CAD build for the part. Positions are in the model's coordinates, mm. A direction names the side the tool comes from. Give positions to 0.01 mm unless a question says otherwise; leave off trailing zeros. Loops run counter-clockwise (first coordinate to the right, second up) from the corner with the lowest first, then second, coordinate; pieces in that order, holes last. Notation, with made-up numbers: (-0.75, 76) - (42.25, 76) arc R33 cw to (42.25, 109) - close; hole circle Ø7 at (74, 21). An arc over 180 degrees is marked (long way). Return JSON: item names as keys, results as strings.
from build123d import *

# Parameters (mm, degrees)
BOSS_EXTRUDE1_DEPTH       = 35
BOSS_EXTRUDE1_DEPTH_BACK  = 35
SKETCH2_W                 = 70
SKETCH2_H                 = 70
BOSS_EXTRUDE2_DEPTH       = 32.5
BOSS_EXTRUDE2_DEPTH_BACK  = 32.5
SKETCH3_W                 = 10
SKETCH3_H                 = 65
BOSS_EXTRUDE10_DEPTH      = 32.5
BOSS_EXTRUDE10_DEPTH_BACK = 32.5
SKETCH20_W                = 10
SKETCH20_H                = 65
SKETCH6_W                 = 65
SKETCH6_H                 = 65
BOSS_EXTRUDE4_DEPTH       = 10
BOSS_EXTRUDE6_DEPTH       = 32.5
BOSS_EXTRUDE6_DEPTH_BACK  = 32.5
SKETCH12_W                = 66.54355119
SKETCH12_H                = 10
SKETCH13_W                = 15
SKETCH13_H                = 15.886543597
BOSS_EXTRUDE7_DEPTH       = 19
BOSS_EXTRUDE7_DEPTH_BACK  = 19
SKETCH16_W                = 15.65
SKETCH16_H                = 15
BOSS_EXTRUDE14_DEPTH      = 65
CUT_EXTRUDE2_REACH        = 292.31
SKETCH25_R                = 3.001207037
SKETCH25_R_2              = 3
CUT_EXTRUDE3_REACH        = 292.31


with BuildPart() as part:
    # Sketch2 → Boss-Extrude1 (new, two sides: drawn at the far end of the back side and taken through both)
    with BuildSketch(Plane.XY.offset(-BOSS_EXTRUDE1_DEPTH_BACK)):
        Rectangle(SKETCH2_W, SKETCH2_H)
    extrude(amount=BOSS_EXTRUDE1_DEPTH + BOSS_EXTRUDE1_DEPTH_BACK)

    # Sketch3 → Boss-Extrude2 (add, two sides: drawn at the far end of the back side and taken through both)
    with BuildSketch(Plane.XY.offset(-BOSS_EXTRUDE2_DEPTH_BACK)):
        with Locations((40, 0)):
            Rectangle(SKETCH3_W, SKETCH3_H)
    extrude(amount=BOSS_EXTRUDE2_DEPTH + BOSS_EXTRUDE2_DEPTH_BACK)

    # Sketch20 → Boss-Extrude10 (add, two sides: drawn at the far end of the back side and taken through both)
    with BuildSketch(Plane.XY.offset(-BOSS_EXTRUDE10_DEPTH_BACK)):
        with Locations((-40, 0)):
            Rectangle(SKETCH20_W, SKETCH20_H)
    extrude(amount=BOSS_EXTRUDE10_DEPTH + BOSS_EXTRUDE10_DEPTH_BACK)

    # Sketch4 → Revolve1 (revolve)
    with BuildSketch(Plane.XY, mode=Mode.PRIVATE) as revolve1_sk:
        Polygon((45, 28), (59.607985015, 28), (59.607985015, 29.5), (67.607985015, 29.5), (74.107985015, 26.85697368), (74.107985015, 0), (45, 0), align=None)
    revolve(revolve1_sk.sketch.rotate(Axis((126.079032841, 0, 0), (-1, 0, 0)), 90), axis=Axis((126.079032841, 0, 0), (-1, 0, 0)))

    # Sketch5 → Revolve2 (revolve)
    with BuildSketch(Plane.XY, mode=Mode.PRIVATE) as revolve2_sk:
        Polygon((74.107985015, 25), (174.107985015, 0), (74.107985015, 0), align=None)
    revolve(revolve2_sk.sketch.rotate(Axis((0, 0, 0), (1, 0, 0)), 90), axis=Axis((0, 0, 0), (1, 0, 0)))

    # Sketch11 → Revolve4 (revolve)
    with BuildSketch(Plane.XY, mode=Mode.PRIVATE) as revolve4_sk:
        Polygon((-45, 28), (-57.201085702, 28), (-57.201085702, 31.288573188), (-80.147769564, 31.288573188), (-80.147769564, 30.339674147), (-106.73557157, 30.339674147), (-106.73557157, 28), (-148.804473643, 28), (-162.901896786, 23.768340348), (-162.901896786, 13.75175022), (-172.176517275, 13.75175022), (-172.176517275, 11.711333713), (-294.985996393, 11.711333713), (-294.985996393, 0), (-45, 0), align=None)
    revolve(revolve4_sk.sketch.rotate(Axis((0, 0, 0), (-1, 0, 0)), 90), axis=Axis((0, 0, 0), (-1, 0, 0)))

    # Sketch6 → Boss-Extrude4 (add)
    with BuildSketch(Plane.XZ.offset(35)):
        Rectangle(SKETCH6_W, SKETCH6_H)
    extrude(amount=BOSS_EXTRUDE4_DEPTH)

    # Sketch12 → Boss-Extrude6 (add, two sides: drawn at the far end of the back side and taken through both)
    with BuildSketch(Plane.XY.offset(-BOSS_EXTRUDE6_DEPTH_BACK)):
        with Locations((0, 40)):
            Rectangle(SKETCH12_W, SKETCH12_H)
    extrude(amount=BOSS_EXTRUDE6_DEPTH + BOSS_EXTRUDE6_DEPTH_BACK)

    # Sketch13 → Revolve5 (revolve)
    with BuildSketch(Plane.XY, mode=Mode.PRIVATE) as revolve5_sk:
        with Locations((7.5, 52.943271799)):
            Rectangle(SKETCH13_W, SKETCH13_H)
    revolve(revolve5_sk.sketch.rotate(Axis((0, 0, 0), (0, 1, 0)), 90), axis=Axis((0, 0, 0), (0, 1, 0)))

    # Sketch14 → Boss-Extrude7 (add, two sides: drawn at the far end of the back side and taken through both)
    with BuildSketch(Plane.XY.offset(-BOSS_EXTRUDE7_DEPTH_BACK)):
        Polygon((-19, 60.650657798), (19, 60.650657798), (19, 66.650657798), (-7.5, 93.150657798), (-19, 93.150657798), align=None)
    extrude(amount=BOSS_EXTRUDE7_DEPTH + BOSS_EXTRUDE7_DEPTH_BACK)

    # Sketch15 → Revolve6 (revolve)
    with BuildSketch(Plane.XY):
        Polygon((-19, 91.400657798), (-25, 91.400657798), (-25, 82.400657798), (-33.5, 82.400657798), (-33.5, 88.400657798), (-71.5, 88.400657798), (-71.5, 86.900657798), (-79.5, 86.900657798), (-79.5, 76.900657798), (-19, 76.900657798), align=None)
    revolve(axis=Axis((23.08157289, 76.900657798, 0), (-1, 0, 0)))

    # Sketch16 → Revolve7 (revolve)
    with BuildSketch(Plane.XY):
        with Locations((-52.825, 7.5)):
            Rectangle(SKETCH16_W, SKETCH16_H)
    revolve(axis=Axis((0, 0, 0), (-1, 0, 0)))

    # Sketch24 → Boss-Extrude14 (add)
    with BuildSketch(Plane.XY.offset(32.5)):
        Polygon((-32.5, -45), (24.068542495, -101.568542495), (31.139610307, -94.497474683), (-18.357864376, -45), align=None)
    extrude(amount=-BOSS_EXTRUDE14_DEPTH)

    # Sketch25 → Cut-Extrude2 (cut, up to next)
    with BuildSketch(Plane(origin=(-38.75, -38.75, 0), x_dir=(0, 0, 1), z_dir=(-0.7071067811865438, -0.7071067811865512, 0)), mode=Mode.PRIVATE) as cut_extrude2_sk1:
        with Locations(Location((0, -83.838834765, 0), (0, 0, 270))):
            Circle(SKETCH25_R)
    cut_extrude2_tool1 = extrude(cut_extrude2_sk1.sketch, amount=-CUT_EXTRUDE2_REACH, mode=Mode.PRIVATE) & part.part
    # Sketch25 → Cut-Extrude2 (cut, up to next)
    with BuildSketch(Plane(origin=(-38.75, -38.75, 0), x_dir=(0, 0, 1), z_dir=(-0.7071067811865438, -0.7071067811865512, 0)), mode=Mode.PRIVATE) as cut_extrude2_sk2:
        with Locations(Location((-14.142135624, -49.696699141, 0), (0, 0, 270))):
            Circle(SKETCH25_R_2)
    cut_extrude2_tool2 = extrude(cut_extrude2_sk2.sketch, amount=-CUT_EXTRUDE2_REACH, mode=Mode.PRIVATE) & part.part
    # Sketch25 → Cut-Extrude2 (cut, up to next)
    with BuildSketch(Plane(origin=(-38.75, -38.75, 0), x_dir=(0, 0, 1), z_dir=(-0.7071067811865438, -0.7071067811865512, 0)), mode=Mode.PRIVATE) as cut_extrude2_sk3:
        with Locations(Location((-14.142135624, -77.980970389, 0), (0, 0, 270))):
            Circle(SKETCH25_R_2)
    cut_extrude2_tool3 = extrude(cut_extrude2_sk3.sketch, amount=-CUT_EXTRUDE2_REACH, mode=Mode.PRIVATE) & part.part
    # Sketch25 → Cut-Extrude2 (cut, up to next)
    with BuildSketch(Plane(origin=(-38.75, -38.75, 0), x_dir=(0, 0, 1), z_dir=(-0.7071067811865438, -0.7071067811865512, 0)), mode=Mode.PRIVATE) as cut_extrude2_sk4:
        with Locations(Location((14.142135624, -49.696699141, 0), (0, 0, 90))):
            Circle(SKETCH25_R_2)
    cut_extrude2_tool4 = extrude(cut_extrude2_sk4.sketch, amount=-CUT_EXTRUDE2_REACH, mode=Mode.PRIVATE) & part.part
    # Sketch25 → Cut-Extrude2 (cut, up to next)
    with BuildSketch(Plane(origin=(-38.75, -38.75, 0), x_dir=(0, 0, 1), z_dir=(-0.7071067811865438, -0.7071067811865512, 0)), mode=Mode.PRIVATE) as cut_extrude2_sk5:
        with Locations(Location((14.142135624, -77.980970389, 0), (0, 0, 90))):
            Circle(SKETCH25_R_2)
    cut_extrude2_tool5 = extrude(cut_extrude2_sk5.sketch, amount=-CUT_EXTRUDE2_REACH, mode=Mode.PRIVATE) & part.part
    add(cut_extrude2_tool1.solids().sort_by_distance((20.533009, -98.033009, 0))[0], mode=Mode.SUBTRACT)
    add(cut_extrude2_tool2.solids().sort_by_distance((-3.609127, -73.890873, -14.142136))[0], mode=Mode.SUBTRACT)
    add(cut_extrude2_tool3.solids().sort_by_distance((16.390873, -93.890873, -14.142136))[0], mode=Mode.SUBTRACT)
    add(cut_extrude2_tool4.solids().sort_by_distance((-3.609127, -73.890873, 14.142136))[0], mode=Mode.SUBTRACT)
    add(cut_extrude2_tool5.solids().sort_by_distance((16.390873, -93.890873, 14.142136))[0], mode=Mode.SUBTRACT)

    # Sketch26 → Cut-Extrude3 (cut, up to next)
    with BuildSketch(Plane(origin=(-38.75, -38.75, 0), x_dir=(0, 0, 1), z_dir=(-0.7071067811865438, -0.7071067811865512, 0)), mode=Mode.PRIVATE) as cut_extrude3_sk1:
        Polygon((-32.5, -48.838834765), (-21.370348691, -78.805078625), (-9.627269044, -88.838834765), (-32.5, -88.838834765), align=None)
    cut_extrude3_tool1 = extrude(cut_extrude3_sk1.sketch, amount=-CUT_EXTRUDE3_REACH, mode=Mode.PRIVATE) & part.part
    # Sketch26 → Cut-Extrude3 (cut, up to next)
    with BuildSketch(Plane(origin=(-38.75, -38.75, 0), x_dir=(0, 0, 1), z_dir=(-0.7071067811865438, -0.7071067811865512, 0)), mode=Mode.PRIVATE) as cut_extrude3_sk2:
        Polygon((32.5, -48.838834765), (21.370348691, -78.805078625), (9.627269044, -88.838834765), (32.5, -88.838834765), align=None)
    cut_extrude3_tool2 = extrude(cut_extrude3_sk2.sketch, amount=-CUT_EXTRUDE3_REACH, mode=Mode.PRIVATE) & part.part
    add(cut_extrude3_tool1.solids().sort_by_distance((15.48251, -92.98251, -26.196672))[0], mode=Mode.SUBTRACT)
    add(cut_extrude3_tool2.solids().sort_by_distance((15.48251, -92.98251, 26.196672))[0], mode=Mode.SUBTRACT)


solid = part.part
1. Cut at A-A, the plane x = -211. Write the cut outline in (y, z).
Values follow:
{"outline": "circle Ø23.42 at (0, 0)"}
2. Cut at B-B, the plane x = 89.5. Write the cut outline in (y, z).
Values follow:
{"outline": "circle Ø42.3 at (0, 0)"}
3. Pull direction Y, two halves, no side cores. Call faces 1 (the face through (-106.736, 27, -9)), 2 (the face through (-13, 93.151, 0)), 3 (the face through (-19, 84, -13)), 4 (the face through (9.717, -80.245, -27.013)): +Y half, -Y half, draft (parallel to the pull), parting line (faces both ways), or undercut.
Values follow:
{"face 1": "draft", "face 2": "+Y half", "face 3": "undercut", "face 4": "-Y half"}
4. Which spindle directions (+Z, -Z, +X, -X, +Y, -Y) get a long thin tool onto all of the face, cutting with end or side? Do faces 5 (the face through (-4, 74, 19)), 6 (the face through (-4, 74, -19)), 7 (the face through (-8, -41, -32.5)), 8 (the face through (-79.5, 77, 0)). Say none if no direction does.
Values follow:
{"face 5": "+Z, +X, -X, +Y", "face 6": "-Z, +X, -X, +Y", "face 7": "-Z, +X, -X, -Y", "face 8": "+Z, -Z, -X, +Y"}
5. Drop flat-ended pins along their axis: P1, Ø8, axis at y = 42, z = 11, coming from the +X side; P2, Ø6, axis at y = 58.5, z = -21, coming from the +X side; P3, Ø3, axis at x = -72, z = -3, coming from the +Y side. Give the stop position or say it passes through.
Values follow:
{"P1": "stops at x = 33.27", "P2": "stops at x = 19", "P3": "stops at y = 88.29"}
6. Drill centre lines: probe 1 along Y at (x, z) = (-14.5, -28); probe 2 along X at (y, z) = (-69.5, -12.5); probe 3 along Y at (x, z) = (-10.5, 23.5). Where is each one in solid material? Low to high.
Values follow:
{"probe 1": "y = -63 to -48.86, -45 to 45", "probe 2": "x = -8 to -2.77, 4.33 to 6.14", "probe 3": "y = -67 to -52.86, -45 to 45"}
